from build123d import *

# Parameters (mm, degrees)
SKETCH1_R           = 3
SKETCH1_R_2         = 1.5
BOSS_EXTRUDE1_DEPTH = 5
SKETCH2_R           = 6
SKETCH2_R_2         = 3
BOSS_EXTRUDE2_DEPTH = 14


with BuildPart() as part:
    # Sketch1 → Boss-Extrude1 (new body)
    with BuildSketch(Plane.XY):
        with BuildLine():
            Line((-9, 10.723805295), (-9, -10.723805295))
            ThreePointArc((-9, -10.723805295), (0, -14), (9, -10.723805295))
            Line((9, -10.723805295), (9, 10.723805295))
            ThreePointArc((9, 10.723805295), (0, 14), (-9, 10.723805295))
        make_face()
        Circle(SKETCH1_R, mode=Mode.SUBTRACT)
        with Locations((-5, 10)):
            Circle(SKETCH1_R_2, mode=Mode.SUBTRACT)
        with Locations((5, 10)):
            Circle(SKETCH1_R_2, mode=Mode.SUBTRACT)
        with Locations((-5, -10)):
            Circle(SKETCH1_R_2, mode=Mode.SUBTRACT)
        with Locations((5, -10)):
            Circle(SKETCH1_R_2, mode=Mode.SUBTRACT)
    extrude(amount=BOSS_EXTRUDE1_DEPTH)

    # Sketch2 → Boss-Extrude2 (add)
    with BuildSketch(Plane.XY.offset(5)):
        Circle(SKETCH2_R)
        Circle(SKETCH2_R_2, mode=Mode.SUBTRACT)
    extrude(amount=BOSS_EXTRUDE2_DEPTH)


solid = part.part
Work out the finished part from the listing and answer in its coordinate system (mm). A direction names the side the tool comes from. Round coordinates to 2 decimals unless told otherwise and drop trailing zeros. Loops run counter-clockwise (first coordinate to the right, second up) from the corner with the lowest first, then second, coordinate; pieces in that order, holes last. Notation, with made-up numbers: (-36, 87) - (1, 87) arc R11 ccw to (1, 92) - close; hole circle Ø6 at (86, 60.5). An arc over 180 degrees is marked (long way). One line per item, written item: value.
Q1. For faces 5 (the cylindrical face through (-6, 0, 12)), 6 (the flat face through (-9, 0, 2)), determine the directions among +Z, -Z, +X, -X, +Y, -Y from which every point of the face is accessible in a straight line to the end or side of a thin tool.
Check values:
face 5: +Z
face 6: +Z, -Z, -X, +Y, -Y
Q2. The mould has two halves that part along X. Classify faces 1 (the flat face through (9, 0, 2)), 2 (the cylindrical face through (-6.2, 9.1, 2.5)), 3 (the cylindrical face through (0, -14, 2)), 4 (the flat face through (-2, -6, 5)): +X half, -X half, draft (parallel to the pull), parting line (faces both ways), or undercut.
Check values:
face 1: +X half
face 2: undercut
face 3: parting line
face 4: draft
Q3. Find section A-A on y = 0. Give the vertices of the cut face in (x, z), and give its area (3 significant figures).
Check values:
outline: (-9, 0) - (-3, 0) - (-3, 19) - (-6, 19) - (-6, 5) - (-9, 5) - close; (3, 0) - (9, 0) - (9, 5) - (6, 5) - (6, 19) - (3, 19) - close
area: 144 mm2
Q4. Find section D-D on x = -5. Give the vertices of the cut face in (y, z), and give its area (3 significant figures).
Check values:
outline: (-13.08, 0) - (-11.5, 0) - (-11.5, 5) - (-13.08, 5) - close; (-8.5, 0) - (8.5, 0) - (8.5, 5) - (3.32, 5) - (3.32, 19) - (-3.32, 19) - (-3.32, 5) - (-8.5, 5) - close; (11.5, 0) - (13.08, 0) - (13.08, 5) - (11.5, 5) - close
area: 194 mm2
Q5. Straight lines are drawn through the part: probe 1 along Y at (x, z) = (-5, 1.2); probe 2 along Y at (x, z) = (0, 11.5); probe 3 along Z at (x, y) = (6.5, -3.75). For each, find the intervals that lie inside material, in ascending order.
Check values:
probe 1: -13.08 to -11.5, -8.5 to 8.5, 11.5 to 13.08
probe 2: -6 to -3, 3 to 6
probe 3: 0 to 5
Q6. Find section B-B on x = 0. Give the vertices of the cut face in (y, z).
Check values:
outline: (-14, 0) - (-3, 0) - (-3, 19) - (-6, 19) - (-6, 5) - (-14, 5) - close; (3, 0) - (14, 0) - (14, 5) - (6, 5) - (6, 19) - (3, 19) - close
Q7. Find section C-C on y = 10. Give the vertices of the cut face in (x, z).
Check values:
outline: (-9, 0) - (-6.5, 0) - (-6.5, 5) - (-9, 5) - close; (-3.5, 0) - (3.5, 0) - (3.5, 5) - (-3.5, 5) - close; (6.5, 0) - (9, 0) - (9, 5) - (6.5, 5) - close
Q8. Each of these flat-tipped pins is pushed along its axis until it touches: pin 1 Ø3 at (x, y) = (2.5, -9) entering from -Z; pin 2 Ø10 at (x, y) = (-3.5, 10.5) entering from +Z; pin 3 Ø1 at (y, z) = (-5.5, 7) entering from -X; pin 4 Ø10 at (x, z) = (2.5, 12) entering from +Y. Where does it stop, or does it pass through?
Check values:
pin 1: z = 0
pin 2: z = 5
pin 3: x = -3.32
pin 4: y = 6
